```python
from build123d import *

# Parameters (mm, degrees)
SKETCH1_R           = 25
SKETCH1_R_2         = 12.5
SKETCH1_R_3         = 2.95
BOSS_EXTRUDE1_DEPTH = 3
SKETCH4_R           = 2.95
BOSS_EXTRUDE3_DEPTH = 17.5
SKETCH5_R           = 1.25
CUT_EXTRUDE2_DEPTH  = 8


with BuildPart() as part:
    # Sketch1 → Boss-Extrude1 (new body)
    with BuildSketch(Plane.XY):
        Circle(SKETCH1_R)
        Circle(SKETCH1_R_2, mode=Mode.SUBTRACT)
        with Locations((0, 18.75)):
            Circle(SKETCH1_R_3, mode=Mode.SUBTRACT)
        with Locations((16.237976321, -9.375)):
            Circle(SKETCH1_R_3, mode=Mode.SUBTRACT)
        with Locations((-16.237976321, -9.375)):
            Circle(SKETCH1_R_3, mode=Mode.SUBTRACT)
    extrude(amount=BOSS_EXTRUDE1_DEPTH)

    # Sketch4 → Boss-Extrude3 (add)
    with BuildSketch(Plane(origin=(0, 0, 0), x_dir=(-1, 0, 0), z_dir=(0, 0, -1))):
        with Locations((16.237976321, -9.375)):
            Circle(SKETCH4_R)
        with Locations((0, 18.75)):
            Circle(SKETCH4_R)
        with Locations((-16.237976321, -9.375)):
            Circle(SKETCH4_R)
    extrude(amount=-BOSS_EXTRUDE3_DEPTH)

    # Sketch5 → Cut-Extrude2 (cut)
    with BuildSketch(Plane.XY.offset(17.5)):
        with Locations((16.237976321, -9.375)):
            Circle(SKETCH5_R)
        with Locations((-16.237976321, -9.375)):
            Circle(SKETCH5_R)
        with Locations((0, 18.75)):
            Circle(SKETCH5_R)
    extrude(amount=-CUT_EXTRUDE2_DEPTH, mode=Mode.SUBTRACT)


solid = part.part
```
Geometry check sheet. Reference: the model listing, model coordinates, mm. A direction names the side the tool comes from. Coordinates: 2 decimals unless noted, no trailing zeros. Write each loop counter-clockwise with the first axis right and the second up, starting at its lowest first coordinate (ties: lowest second). Pieces come first, ordered by that corner, then holes. Notation, with made-up numbers: M 62,7 L 108,7 A22 ccw 108,45 Z; hole C 23.5,-23 d1. An arc over 180 degrees is marked long. Use one line per item in the form item = value. Start each with the question number.
1) Section check D-D on z = 2. Enter the section's corners in (x, y).
2) Thickness scan on probe 1 along Y at (x, z) = (0, 1.7); probe 2 along Y at (x, z) = (0, 15.25); probe 3 along Z at (x, y) = (8, 13.5). Record the ranges inside material, lowest first. Write a range as from..to.
3) Set-up check for faces 1 (the flat face through (0, 17, 17.5)), 2 (the cylindrical face through (-13.29, -9.25, 10.15)): record each of +Z, -Z, +X, -X, +Y, -Y from which the full face is reachable in a straight line by a thin tool's end or side.
4) Release check for a two-part mould opening along Y. For faces 3 (the flat face through (-11.5, 5.9, 0)), 4 (the cylindrical face through (23.846, 7.509, 1.479)), 5 (the cylindrical face through (16.075, -8.136, 13.556)), 6 (the cylindrical face through (11.923, 3.755, 1.479)) record: pulls with the +Y half, pulls with the -Y half, needs draft (parallel to the pull), parting line crosses it, or undercut.
5) Section check C-C on z = 14.5. Enter the section's corners in (x, y) (3 decimals).
6) Section check A-A on x = 0. Enter the section's corners in (y, z).
7) Go/stop test with flat-tipped pins: pin 1 Ø0.8 at (x, y) = (-0.5, 19) entering from +Z; pin 2 Ø1 at (x, y) = (16, 3.5) entering from +Z; pin 3 Ø3 at (x, z) = (-3, 8) entering from -Y. Record where each tip stops, or that it passes through.
8) Section check B-B on y = 0. Enter the section's corners in (x, z).
Responses:
q1.outline = C 0,0 d50; hole C 0,0 d25
q2.probe_1 = -25..-12.5, 12.5..25
q2.probe_2 = 15.8..17.5, 20..21.7
q2.probe_3 = 0..3
q3.face_1 = +Z, +X, -X, +Y, -Y
q3.face_2 = +Z
q4.face_3 = needs draft
q4.face_4 = parting line crosses it
q4.face_5 = undercut
q4.face_6 = undercut
q5.outline = C -16.238,-9.375 d5.9; C 0,18.75 d5.9; C 16.238,-9.375 d5.9; hole C -16.238,-9.375 d2.5; hole C 0,18.75 d2.5; hole C 16.238,-9.375 d2.5
q6.outline = M -25,0 L -12.5,0 L -12.5,3 L -25,3 Z; M 12.5,0 L 25,0 L 25,3 L 21.7,3 L 21.7,17.5 L 20,17.5 L 20,9.5 L 17.5,9.5 L 17.5,17.5 L 15.8,17.5 L 15.8,3 L 12.5,3 Z
q7.pin_1 = 9.5
q7.pin_2 = 3
q7.pin_3 = 16.21
q8.outline = M -25,0 L -12.5,0 L -12.5,3 L -25,3 Z; M 12.5,0 L 25,0 L 25,3 L 12.5,3 Z
